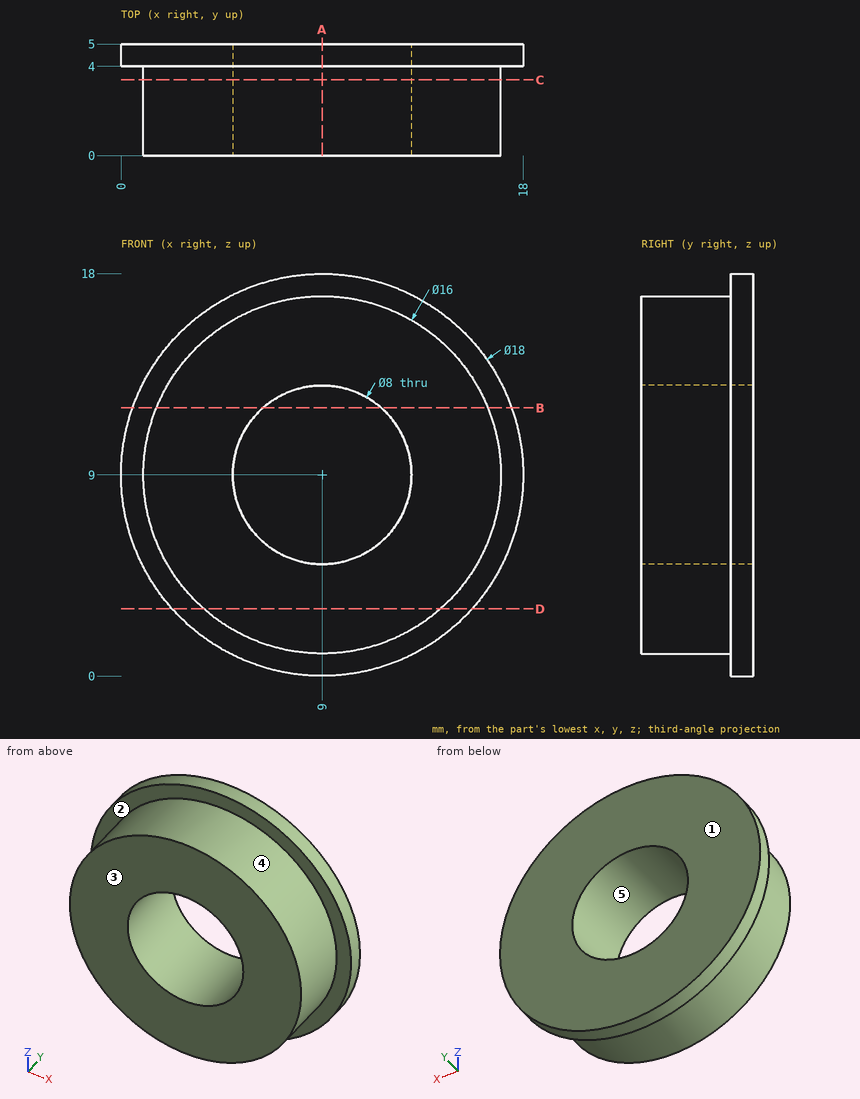
Geometry check sheet. Reference: drawing and pictorial views, mm from the part's lowest x, y, z. A direction names the side the tool comes from. Round coordinates to 2 decimals unless told otherwise and drop trailing zeros. Loops run counter-clockwise (first coordinate to the right, second up) from the corner with the lowest first, then second, coordinate; pieces in that order, holes last. Notation, with made-up numbers: (47.25, 80.5) - (51.25, 80.5) arc R8 cw to (51.25, 84.5) - close; hole circle Ø6 at (-13.75, -33.5). An arc over 180 degrees is marked (long way). Write item = value, one per line. Start each with the question number.
Q1. Access from +Z, -Z, +X, -X, +Y, -Y to the whole of each face (thin tool, end or side, straight path). Record for the marked faces 1 and 2.
Q2. Section check B-B (z = 12). Record the boundary of the cut face in (x, y), plus the area to 3 significant figures.
Q3. Section check D-D (z = 3). Record the boundary of the cut face in (x, y), plus the area to 3 significant figures.
Q4. Release check for a two-part mould opening along Z. For the marked faces 3, 4 and 5 record: pulls with the +Z half, pulls with the -Z half, needs draft (parallel to the pull), parting line crosses it, or undercut.
Q5. Section check A-A (x = 9). Record the boundary of the cut face in (y, z), plus the area to 3 significant figures.
Q6. Depth check by flat-ended pin: P1, Ø1.5, axis at x = 6, y = 3.5, coming from the +Z side. Enter the tip coordinate at first touch or a pass-through.
Q7. Section check C-C (y = 3.4). Record the boundary of the cut face in (x, z), plus the area to 3 significant figures.
Q8. Thickness scan on L1, parallel to Z at x = 9, y = 2.6; L2, parallel to X at y = 4.05, z = 9. Record the ranges inside material, lowest first.
Derived:
q1.face_1 = +Z, -Z, +X, -X, +Y
q1.face_2 = -Y
q2.outline = (0.51, 4) - (1.58, 4) - (1.58, 0) - (6.35, 0) - (6.35, 5) - (0.51, 5) - close; (11.65, 0) - (16.42, 0) - (16.42, 4) - (17.49, 4) - (17.49, 5) - (11.65, 5) - close
q2.area = 49.8 mm^2
q3.outline = (2.29, 4) - (3.71, 4) - (3.71, 0) - (14.29, 0) - (14.29, 4) - (15.71, 4) - (15.71, 5) - (2.29, 5) - close
q3.area = 55.7 mm^2
q4.face_3 = needs draft
q4.face_4 = parting line crosses it
q4.face_5 = undercut
q5.outline = (0, 1) - (4, 1) - (4, 0) - (5, 0) - (5, 5) - (0, 5) - close; (0, 13) - (5, 13) - (5, 18) - (4, 18) - (4, 17) - (0, 17) - close
q5.area = 42.0 mm^2
q6.P1 = 17.66
q7.outline = circle Ø16 at (9, 9); hole circle Ø8 at (9, 9)
q7.area = 151 mm^2
q8.L1 = 1 to 5, 13 to 17
q8.L2 = 0 to 5, 13 to 18
